```python
from build123d import *

# Parameters (mm, degrees)
SKETCH_1_R      = 1.5
EXTRUDE_1_DEPTH = 3
SKETCH_3_W      = 5
SKETCH_3_H      = 12
EXTRUDE_2_DEPTH = 3
SKETCH_4_R      = 1.5
EXTRUDE_3_DEPTH = 3


with BuildPart() as part:
    # 草图1 → 凸台-拉伸1 (new body)
    with BuildSketch(Plane(origin=(0, 0, 0), x_dir=(1, 0, 0), z_dir=(0, 1, 0))):
        Polygon((-2.5, -1.5), (-2.5, -10.5), (2.5, -10.5), (2.5, 10.5), (-2.5, 10.5), (-2.5, 1.5), (-6.5, 1.5), (-6.5, -1.5), align=None)
        with Locations(Location((0, 8, 0), (0, 0, 270))):
            Circle(SKETCH_1_R, mode=Mode.SUBTRACT)
        with Locations(Location((0, -8, 0), (0, 0, 270))):
            Circle(SKETCH_1_R, mode=Mode.SUBTRACT)
    extrude(amount=EXTRUDE_1_DEPTH)

    # 草图3 → 凸台-拉伸2 (add)
    with BuildSketch(Plane(origin=(0, 3, 0), x_dir=(1, 0, 0), z_dir=(0, 1, 0))):
        with Locations((0, 16.5)):
            Rectangle(SKETCH_3_W, SKETCH_3_H)
        with Locations((0, -16.5)):
            Rectangle(SKETCH_3_W, SKETCH_3_H)
    extrude(amount=-EXTRUDE_2_DEPTH)

    # 草图4 → 凸台-拉伸3 (add)
    with BuildSketch(Plane(origin=(0, 0, -22.5), x_dir=(-1, 0, 0), z_dir=(0, 0, -1))):
        with BuildLine():
            Line((-2.5, 3), (-13.5, 3))
            ThreePointArc((-13.5, 3), (-14.207106781, 2.707106781), (-14.5, 2))
            Line((-14.5, 2), (-14.5, -2))
            ThreePointArc((-14.5, -2), (-14.207106781, -2.707106781), (-13.5, -3))
            Line((-13.5, -3), (-10.5, -3))
            ThreePointArc((-10.5, -3), (-9.792893219, -2.707106781), (-9.5, -2))
            Line((-9.5, -2), (-9.5, -1))
            ThreePointArc((-9.5, -1), (-9.207106781, -0.292893219), (-8.5, 0))
            Line((-8.5, 0), (-2.5, 0))
            Line((-2.5, 0), (-2.5, 3))
        make_face()
        with Locations((-12, -1)):
            Circle(SKETCH_4_R, mode=Mode.SUBTRACT)
    extrude_3 = extrude(amount=-EXTRUDE_3_DEPTH)

    # 镜向1: 凸台-拉伸3 across plane
    add(extrude_3.mirror(Plane.XY))


solid = part.part
```
Work out the finished part from the listing and answer in its coordinate system (mm). A direction names the side the tool comes from. Coordinates: 2 decimals unless noted, no trailing zeros. Write each loop counter-clockwise with the first axis right and the second up, starting at its lowest first coordinate (ties: lowest second). Pieces come first, ordered by that corner, then holes. Notation, with made-up numbers: (-23, -22) - (-7, -22) arc R14 cw to (-7, -14) - close; hole circle Ø1 at (16, -13). An arc over 180 degrees is marked (long way). Answer as a JSON object with one key per item and string values.
Q1. Given pin 1 Ø1.8 at (x, z) = (0, 8) entering from -Y; pin 2 Ø1.1 at (y, z) = (-1.5, -21.5) entering from -X; pin 3 Ø3.5 at (x, z) = (0, -8) entering from -Y; pin 4 Ø1.5 at (y, z) = (1, -6) entering from +X, each flat-ended and moving along its own axis, determine where each tip first touches the part or whether it passes through.
Results list:
{"pin 1": "passes through", "pin 2": "stops at x = 9.5", "pin 3": "stops at y = 0", "pin 4": "stops at x = 2.5"}
Q2. Which of the six approach directions +Z, -Z, +X, -X, +Y, -Y give full straight-line access (tool end or side, diameter ignored) to faces 1 (the flat face through (9.5, -1.5, 21)), 2 (the flat face through (-5, 1, 1.5)), 3 (the flat face through (-2.5, 2, -12)), 4 (the flat face through (2.5, 2, 0)), 5 (the flat face through (6, 1, 22.5))?
Results list:
{"face 1": "+Z, -Z, -X, -Y", "face 2": "+Z, -X, +Y, -Y", "face 3": "-Z, -X, +Y, -Y", "face 4": "+X, +Y, -Y", "face 5": "+Z, +X, -X, +Y, -Y"}
Q3. Find section C-C (x = 4.25). Write down the section's boundary in (y, z), plus the area to 3 significant figures.
Results list:
{"outline": "(0, -22.5) - (3, -22.5) - (3, -19.5) - (0, -19.5) - close; (0, 19.5) - (3, 19.5) - (3, 22.5) - (0, 22.5) - close", "area": "18.0 mm^2"}
Q4. Find section A-A (x = 0). Write down the section's boundary in (y, z), plus the area to 3 significant figures.
Results list:
{"outline": "(0, -22.5) - (3, -22.5) - (3, -9.5) - (0, -9.5) - close; (0, -6.5) - (3, -6.5) - (3, 6.5) - (0, 6.5) - close; (0, 9.5) - (3, 9.5) - (3, 22.5) - (0, 22.5) - close", "area": "117 mm^2"}
Q5. Consider L1, parallel to Z at x = 4.75, y = 0.3; L2, parallel to Y at x = 12, z = 21.4; L3, parallel to X at y = 1.35, z = -8. Determine where each line is inside the solid, lowest interval first. Write a range as from..to.
Results list:
{"L1": "z = -22.5..-19.5, 19.5..22.5", "L2": "y = -3..-2.5, 0.5..3", "L3": "x = -2.5..-1.5, 1.5..2.5"}
Q6. For a pull along X with two mould halves and no side action, classify faces 6 (the flat face through (14.5, 0, 21)), 7 (the flat face through (9, 1, 19.5)), 8 (the cylindrical face through (0.07, 1.48, 6.5)) as pulls with the +X half, pulls with the -X half, needs draft (parallel to the pull), parting line crosses it, or undercut.
Results list:
{"face 6": "pulls with the +X half", "face 7": "needs draft", "face 8": "undercut"}
Q7. Find section B-B (z = 8). Write down the section's boundary in (x, y).
Results list:
{"outline": "(-2.5, 0) - (-1.5, 0) - (-1.5, 3) - (-2.5, 3) - close; (1.5, 0) - (2.5, 0) - (2.5, 3) - (1.5, 3) - close"}
Q8. Find section D-D (y = 1.55). Write down the section's boundary in (x, z), plus the area to 3 significant figures.
Results list:
{"outline": "(-6.5, -1.5) - (-2.5, -1.5) - (-2.5, -22.5) - (14.5, -22.5) - (14.5, -19.5) - (2.5, -19.5) - (2.5, 19.5) - (14.5, 19.5) - (14.5, 22.5) - (-2.5, 22.5) - (-2.5, 1.5) - (-6.5, 1.5) - close; hole circle Ø3 at (0, -8); hole circle Ø3 at (0, 8)", "area": "295 mm^2"}
